Can you work these out from the model? Positions are in its coordinate system, mm. Give positions to 0.01 mm unless a question says otherwise; leave off trailing zeros. Loops run counter-clockwise (first coordinate to the right, second up) from the corner with the lowest first, then second, coordinate; pieces in that order, holes last. Notation, with made-up numbers: M 78.5,-3.75 L 88.5,-3.75 A15 ccw 88.5,11.25 Z; hole C -30,29.5 d9. An arc over 180 degrees is marked long. Put each result on its own line as item: value. Start each with the question number.
1) Imagine slicing it at C-C (y = -26.5). Write out the boundary of the cut face in (x, z).
2) Imagine slicing it at A-A (x = 0). Write out the boundary of the cut face in (y, z), then the cut area to 3 significant figures.
3) Imagine slicing it at D-D (x = 26). Write out the boundary of the cut face in (y, z), then the cut area to 3 significant figures.
4) Imagine slicing it at B-B (z = 1.6). State how many separate pieces and enclosed holes the cut face has, then the cut area to 3 significant figures.
5) For P1, Ø0.9, axis at x = 56.5, z = 1.5, coming from the +Y side; P2, Ø3.5, axis at x = 60, y = 45, coming from the +Z side; P3, Ø0.5, axis at x = 13, z = -0.5, coming from the -Y side; P4, Ø0.8, axis at y = 60.5, z = -0.5, coming from the -X side, each with a flat end and sliding along its axis, tell me the tip position at first contact or that it passes through.
6) Please list where these lines run through material, in increasing order: line 1 along Y through (x, z) = (0, 1.8); line 2 along Y through (x, z) = (75, 2.3); line 3 along Z through (x, y) = (-32.5, -42.5). Write a range as from..to.
from build123d import *

# Parameters (mm, degrees)
SKETCH1_R           = 10.5
SKETCH1_R_2         = 8
BOSS_EXTRUDE1_DEPTH = 3
CUT_EXTRUDE1_REACH  = 140.687
SKETCH2_R           = 2
BOSS_EXTRUDE2_DEPTH = 3
SKETCH4_W           = 2
SKETCH4_H           = 6.5
SKETCH4_W_2         = 6.5
SKETCH4_H_2         = 2
BOSS_EXTRUDE3_DEPTH = 1
SKETCH5_R           = 2
CUT_EXTRUDE2_DEPTH  = 10


with BuildPart() as part:
    # Sketch1 → Boss-Extrude1 (new body)
    # profile 1 of 2: a face of its own
    with BuildSketch(Plane.XY):
        with BuildLine():
            ThreePointArc((-60, 0), (-52.867640737, 28.372743309), (-33.166247904, 50))
            Line((-33.166247904, 50), (-60, 50))
            Line((-60, 50), (-60, 0))
        make_face()
    # profile 2 of 2: a face of its own
    with BuildSketch(Plane.XY):
        with BuildLine():
            ThreePointArc((0, 60), (-17.320508076, 57.445626465), (-33.166247904, 50))
            ThreePointArc((-33.166247904, 50), (-52.867640737, 28.372743309), (-60, 0))
            ThreePointArc((-60, 0), (-6.678621673, -59.627141576), (58.513200418, -13.274237334))
            Line((58.513200418, -13.274237334), (87.081101726, -13.274237334))
            Line((87.081101726, -13.274237334), (117.67766953, 17.32233047))
            ThreePointArc((117.67766953, 17.32233047), (123.096988313, 44.567085809), (100, 60))
            Line((100, 60), (0, 60))
        make_face()
        Circle(SKETCH1_R, mode=Mode.SUBTRACT)
        with Locations((100, 35)):
            Circle(SKETCH1_R_2, mode=Mode.SUBTRACT)
    extrude(amount=BOSS_EXTRUDE1_DEPTH)

    # Sketch2 → Cut-Extrude1 (cut, up to next)
    with BuildSketch(Plane.XY.offset(3), mode=Mode.PRIVATE) as cut_extrude1_sk1:
        with Locations((60, 45)):
            Circle(SKETCH2_R)
    cut_extrude1_tool1 = extrude(cut_extrude1_sk1.sketch, amount=-CUT_EXTRUDE1_REACH, mode=Mode.PRIVATE) & part.part
    # Sketch2 → Cut-Extrude1 (cut, up to next)
    with BuildSketch(Plane.XY.offset(3), mode=Mode.PRIVATE) as cut_extrude1_sk2:
        with Locations((75, 11.725762666)):
            Circle(SKETCH2_R)
    cut_extrude1_tool2 = extrude(cut_extrude1_sk2.sketch, amount=-CUT_EXTRUDE1_REACH, mode=Mode.PRIVATE) & part.part
    add(cut_extrude1_tool1.solids().sort_by_distance((60, 45, 3))[0], mode=Mode.SUBTRACT)
    add(cut_extrude1_tool2.solids().sort_by_distance((75, 11.725763, 3))[0], mode=Mode.SUBTRACT)

    # Sketch3 → Boss-Extrude2 (add)
    with BuildSketch(Plane(origin=(0, 0, 0), x_dir=(-1, 0, 0), z_dir=(0, 0, -1))):
        with BuildLine():
            Line((-30, 80), (-30, 60))
            Line((-30, 60), (0, 60))
            ThreePointArc((0, 60), (2.502176759, 59.947803225), (5, 59.791303716))
            Line((5, 59.791303716), (5, 80))
            Line((5, 80), (-30, 80))
        make_face()
    extrude(amount=-BOSS_EXTRUDE2_DEPTH)

    # Sketch4 → Boss-Extrude3 (add)
    with BuildSketch(Plane(origin=(0, 0, 0), x_dir=(-1, 0, 0), z_dir=(0, 0, -1))):
        with Locations((-12.5, 68.846087829)):
            Rectangle(SKETCH4_W, SKETCH4_H)
        with Locations((-16.75, 64.596087829)):
            Rectangle(SKETCH4_W_2, SKETCH4_H_2)
        with Locations((-12.5, 64.596087829)):
            Rectangle(SKETCH4_W, SKETCH4_H_2)
        with Locations((-8.25, 64.596087829)):
            Rectangle(SKETCH4_W_2, SKETCH4_H_2)
        with Locations((-12.5, 60.346087829)):
            Rectangle(SKETCH4_W, SKETCH4_H)
    extrude(amount=BOSS_EXTRUDE3_DEPTH)

    # Sketch5 → Cut-Extrude2 (cut)
    with BuildSketch(Plane.XY.offset(3)):
        with Locations((92, 43)):
            Circle(SKETCH5_R)
        with Locations((108, 43)):
            Circle(SKETCH5_R)
        with Locations((108, 27)):
            Circle(SKETCH5_R)
        with Locations((92, 27)):
            Circle(SKETCH5_R)
    extrude(amount=-CUT_EXTRUDE2_DEPTH, mode=Mode.SUBTRACT)


solid = part.part
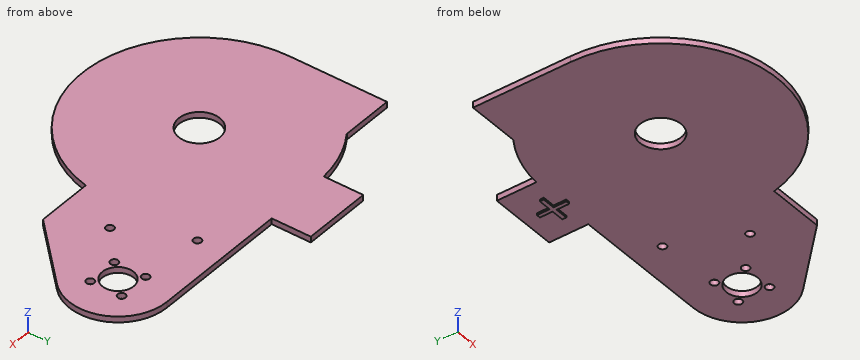
Recorded:
1. outline: M -53.83,0 L 53.83,0 L 53.83,3 L -53.83,3 Z
2. outline: M -60,0 L -10.5,0 L -10.5,3 L -60,3 Z; M 10.5,0 L 80,0 L 80,3 L 10.5,3 Z
2. area: 357 mm²
3. outline: M -54.07,0 L 80,0 L 80,3 L -54.07,3 Z
3. area: 402 mm²
4. separate pieces: 1
4. enclosed holes: 8
4. area: 16,500 mm²
5. P1: y = 60
5. P2: through
5. P3: y = 57.1
5. P4: x = 11.5
6. line 1: -60..-10.5, 10.5..80
6. line 2: -13.27..9.73, 13.73..60
6. line 3: 0..3
